from build123d import *

# Parameters (mm, degrees)
SKETCH_1_W          = 20
SKETCH_1_H          = 20
SKETCH_1_R          = 1.75
EXTRUDE_1_DEPTH     = 3
SKETCH_2_W          = 20
SKETCH_2_H          = 3
EXTRUDE_2_DEPTH     = 17
SKETCH_3_R          = 1.75
CUT_EXTRUDE_1_DEPTH = 17
EXTRUDE_4_DEPTH     = 3
EXTRUDE_5_DEPTH     = 3


with BuildPart() as part:
    # Эскиз1 → Бобышка-Вытянуть1 (new body)
    with BuildSketch(Plane(origin=(0, 0, 0), x_dir=(1, 0, 0), z_dir=(0, 1, 0))):
        Rectangle(SKETCH_1_W, SKETCH_1_H)
        with Locations(Location((0, 0, 0), (0, 0, 270))):
            Circle(SKETCH_1_R, mode=Mode.SUBTRACT)
    extrude(amount=EXTRUDE_1_DEPTH)

    # Эскиз2 → Бобышка-Вытянуть2 (add)
    with BuildSketch(Plane(origin=(0, 3, 0), x_dir=(1, 0, 0), z_dir=(0, 1, 0))):
        with Locations((0, 8.5)):
            Rectangle(SKETCH_2_W, SKETCH_2_H)
    extrude(amount=EXTRUDE_2_DEPTH)

    # Эскиз3 → Вырез-Вытянуть1 (cut)
    with BuildSketch(Plane.XY.offset(-7)):
        with Locations((0, 10)):
            Circle(SKETCH_3_R)
    extrude(amount=-CUT_EXTRUDE_1_DEPTH, mode=Mode.SUBTRACT)

    # Эскиз4 → Бобышка-Вытянуть4 (add)
    with BuildSketch(Plane.ZY.offset(10)):
        Polygon((-7, 20), (10, 3), (-7, 3), align=None)
    extrude(amount=-EXTRUDE_4_DEPTH)

    # Эскиз5 → Бобышка-Вытянуть5 (add)
    with BuildSketch(Plane(origin=(10, 0, 0), x_dir=(0, 0, -1), z_dir=(1, 0, 0))):
        Polygon((7, 20), (7, 3), (-10, 3), align=None)
    extrude(amount=-EXTRUDE_5_DEPTH)


solid = part.part
The model under review builds one solid part; all positions refer to its coordinate system, in mm. A direction names the side the tool comes from. Round coordinates to 2 decimals unless told otherwise and drop trailing zeros. Order: outer loops, then holes, each group sorted by start corner. A loop starts at its lowest first (then second) coordinate and runs counter-clockwise, first axis right, second up. Notation, with made-up numbers: (37.25, 59) -> (89.25, 59) arc R5 ccw to (89.25, 68) -> close; hole circle Ø1 at (3.5, 52.5). An arc over 180 degrees is marked (long way). Use CSV: the item, a comma, the result in double quotes. Start each with the question number.
(1) Wall thickness on probe 1 along Y at (x, z) = (0, -9.05); probe 2 along X at (y, z) = (1.5, 0); probe 3 along X at (y, z) = (13, -6.5): over which ranges is each line inside the solid? List them lowest first. Write a range as from..to.
(2) Consider section C-C on x = -0.5. Write out the cut boundary in (y, z).
(3) Insertion check: pin 1 (4 mm diameter, centred on x = -6.5, z = -2, fed in from +Y); pin 2 (5.5 mm diameter, centred on x = 0, y = 10, fed in from +Z); pin 3 (3 mm diameter, centred on x = -1.5, z = 7.5, fed in from +Y). Each pin has a flat end and moves straight along its axis. Give the tip position at first contact, or say it passes through.
(4) Tool access review of faces 1 (the face through (0, 20, -9)), 2 (the face through (-7, 8, -2)): name each direction out of +Z, -Z, +X, -X, +Y, -Y from which nothing blocks a thin tool from reaching the whole face with its end or side.
(5) Consider section B-B on z = 0. Write out the cut boundary in (x, y).
(6) Consider section A-A on y = 10. Write out the cut boundary in (x, z).
(7) Consider section D-D on y = 18. Write out the cut boundary in (x, z).
(8) Mouldability with a two-part tool opening along X and no side actions: class faces 3 (the face through (9, 11, 2)), 4 (the face through (-1.71, 1.48, -0.38)), 5 (the face through (-10, 8, -2)) as pulls with the +X half, pulls with the -X half, needs draft (parallel to the pull), parting line crosses it, or undercut.
Responses:
1,probe 1,"0..8.25, 11.75..20"
1,probe 2,"-10..-1.75, 1.75..10"
1,probe 3,"-10..-7, 7..10"
2,outline,"(0, -10) -> (8.32, -10) -> (8.32, -7) -> (3, -7) -> (3, -1.68) -> (0, -1.68) -> close; (0, 1.68) -> (3, 1.68) -> (3, 10) -> (0, 10) -> close; (11.68, -10) -> (20, -10) -> (20, -7) -> (11.68, -7) -> close"
3,pin 1,"y = 16.94"
3,pin 2,"z = -7"
3,pin 3,"y = 3"
4,face 1,"+Z, -Z, +X, -X, +Y"
4,face 2,"+Z, +Y"
5,outline,"(-10, 0) -> (-1.75, 0) -> (-1.75, 3) -> (-7, 3) -> (-7, 13) -> (-10, 13) -> close; (1.75, 0) -> (10, 0) -> (10, 13) -> (7, 13) -> (7, 3) -> (1.75, 3) -> close"
6,outline,"(-10, -10) -> (-1.75, -10) -> (-1.75, -7) -> (-7, -7) -> (-7, 3) -> (-10, 3) -> close; (1.75, -10) -> (10, -10) -> (10, 3) -> (7, 3) -> (7, -7) -> (1.75, -7) -> close"
7,outline,"(-10, -10) -> (10, -10) -> (10, -5) -> (7, -5) -> (7, -7) -> (-7, -7) -> (-7, -5) -> (-10, -5) -> close"
8,face 3,"needs draft"
8,face 4,"undercut"
8,face 5,"pulls with the -X half"
